Design review of the part built by this model. Coordinates are the model's own, in mm. Face numbers are marked on the shaded views. A direction names the side the tool comes from. Coordinates: 2 decimals unless noted, no trailing zeros. Write each loop counter-clockwise with the first axis right and the second up, starting at its lowest first coordinate (ties: lowest second). Pieces come first, ordered by that corner, then holes. Notation, with made-up numbers: (-18.5, -7.75) - (29.5, -7.75) arc R24 ccw to (29.5, 16.25) - close; hole circle Ø5 at (82, -18). An arc over 180 degrees is marked (long way). Answer as a JSON object with one key per item and string values.
Autodesk Inventor part; units mm, degrees
ref_plane "YZ Plane" through (0, 0, 0) normal (1, 0, 0) x (0, 1, 0)
ref_plane "XZ Plane" through (0, 0, 0) normal (0, 1, 0) x (-1, 0, 0)
ref_plane "XY Plane" through (0, 0, 0) normal (0, 0, 1) x (1, 0, 0)
sketch "Sketch1" plane through (0, 0, 0) normal (0, 0, 1) x (1, 0, 0)
  point P0 (0, 0)
sketch "Sketch2" plane through (0, 0, 0) normal (0, 1, 0) x (-1, 0, 0)
  line L0 (11.1114, 10.1278) -> (-7.2886, 10.1278)
  line L1 (-7.2886, 10.1278) -> (-7.2886, -10.8722)
  line L2 (-7.2886, -10.8722) -> (11.1114, -10.8722)
  line L3 (11.1114, -10.8722) -> (11.1114, 10.1278)
  point P0 (0, 0)
  dimension "d0" = 21
  dimension "d1" = 18.4
extrude "Extrusion1" add sketch "Sketch2" along normal blind 0.5
sketch "Sketch3" plane through (0, 0.5, 0) normal (0, 1, 0) x (1, 0, 0)
  circle A0 centre (-1.9114, -0.9278) radius 9.2
  line L0 (-11.1114, -10.1278) -> (7.2886, -10.1278)
  line L1 (7.2886, -10.1278) -> (7.2886, 10.8722)
  line L2 (7.2886, -10.1278) -> (7.2886, 10.8722)
  line L3 (7.2886, 10.8722) -> (-11.1114, 10.8722)
  line L4 (-11.1114, 10.8722) -> (-11.1114, -10.1278)
  line L5 (-11.1114, -10.1278) -> (7.2886, -10.1278)
  point P0 (0, 0)
  point P1 (-11.1114, -0.9278)
  point P2 (7.2886, -0.9278)
  dimension "d4" = 18.4
extrude "Extrusion2" add sketch "Sketch3" along normal blind 1 contours A0 | A0 L4 L3 L1
sketch "Sketch6" plane through (-11.1114, 0, -10.8722) normal (-1, 0, 0) x (0, 0, 1)
  line L0 (0, 0) -> (21, 0)
  line L1 (21, 0) -> (21, 0.5)
  line L2 (11.8, 0.5) -> (21, 0.5)
  line L3 (11.8, 0.5) -> (11.8, 1.5)
  line L4 (0, 1.5) -> (11.8, 1.5)
  line L5 (0, 0) -> (0, 1.5)
  line L6 (11.8, 0.5) -> (0, 0.75)
  point P0 (10.8722, 0)
extrude "Extrusion4" add sketch "Sketch6" along normal blind 3 contours L5 L6 L2 L1 L0
sketch "Sketch7" plane through (-14.1114, 0, -10.8722) normal (-1, 0, 0) x (0, 0, 1)
  line L0 (0, 0) -> (0, 1.5)
  line L1 (0, 0.75) -> (0, -0.116)
  line L2 (0, -0.116) -> (21, -0.116)
  line L3 (0, 0) -> (21, 0)
  line L4 (21, -0.116) -> (21, 0)
  point P0 (10.8722, 0)
  dimension "d11" = 0.866
extrude "Extrusion5" add sketch "Sketch7" against normal up to surface (21.4 mm away)
properties part number "klapka"
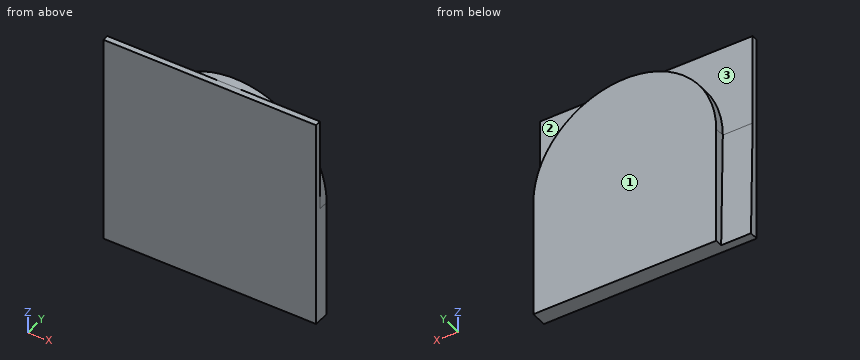
(1) Take a section at B-B, the plane y = 1. Write out the cut boundary in (x, z), and give its area (3 significant figures).
Solved:
{"outline": "(-11.11, -10.87) - (7.29, -10.87) - (7.29, 0.93) arc R9.2 ccw to (-11.11, 0.93) - close", "area": "350 mm^2"}
(2) For pin 1 (0.5 mm diameter, centred on y = 1, z = -5.5, fed in from -X), flat-tipped, find the tip position at first contact; note if it passes through.
Solved:
{"pin 1": "stops at x = -11.11"}
(3) Take a section at C-C, the plane x = -8. Write out the cut boundary in (y, z), and give its area (3 significant figures).
Solved:
{"outline": "(-0.12, -10.87) - (1.5, -10.87) - (1.5, 7.82) - (0.5, 7.82) - (0.5, 10.13) - (-0.12, 10.13) - close", "area": "31.6 mm^2"}
(4) Take a section at A-A, the plane z = 6.5. Write out the cut boundary in (x, y), and give its area (3 significant figures).
Solved:
{"outline": "(-14.11, -0.12) - (7.29, -0.12) - (7.29, 0.5) - (5.41, 0.5) - (5.41, 1.5) - (-9.23, 1.5) - (-9.23, 0.5) - (-14.11, 0.5) - close", "area": "27.8 mm^2"}
(5) Take a section at D-D, the plane z = -8. Write out the cut boundary in (x, y), and give its area (3 significant figures).
Solved:
{"outline": "(-14.11, -0.12) - (7.29, -0.12) - (7.29, 1.5) - (-11.11, 1.5) - (-11.11, 0.69) - (-14.11, 0.69) - close", "area": "32.1 mm^2"}
(6) To check wall thickness, follow line 1 (Y direction, x = -11.75, z = 6); line 2 (X direction, y = 0.8, z = -2.5); line 3 (Z direction, x = -1.75, y = 1). State the ranges of each line that lie inside material, in increasing order. Write a range as from..to.
Solved:
{"line 1": "y = -0.12..0.5", "line 2": "x = -11.11..7.29", "line 3": "z = -10.87..10.13"}
(7) Tool access review of the marked faces 1, 2 and 3: name each direction out of +Z, -Z, +X, -X, +Y, -Y from which nothing blocks a thin tool from reaching the whole face with its end or side.
Solved:
{"face 1": "+Z, -Z, +X, -X, +Y", "face 2": "+Z, +X, +Y", "face 3": "+Z, -X, +Y"}
